Answer from the drawing. Dimensions are ordinates in mm from the lowest x, y and z of the part. A direction names the side the tool comes from. Round coordinates to 2 decimals unless told otherwise and drop trailing zeros. Write each loop counter-clockwise with the first axis right and the second up, starting at its lowest first coordinate (ties: lowest second). Pieces come first, ordered by that corner, then holes.
1. Find section C-C (y = 5.75). Write down the section's boundary in (x, z) (3 decimals).
2. Find section D-D (y = 23.75). Write down the section's boundary in (x, z) (3 decimals), and give its area (3 significant figures).
3. Find section B-B (z = 14). Write down the section's boundary in (x, y), and give its area (3 significant figures).
4. Determine the mould class of the marked faces 3, 4 and 5 for opening direction Z: pulls with the +Z half, pulls with the -Z half, needs draft (parallel to the pull), parting line crosses it, or undercut.
5. Straight lines are drawn through the part: probe 1 along Y at (x, z) = (18, 2); probe 2 along X at (y, z) = (14.5, 16.5); probe 3 along Z at (x, y) = (16, 20). For each, find the intervals that lie inside material, in ascending order.
6. A tool of negligible diameter and unlimited length cuts with its end or side. For the marked faces 1 and 2, from which of +Z, -Z, +X, -X, +Y, -Y can it reach the whole face along a straight path? Write none if from no direction.
7. Find section A-A (x = 22). Write down the section's boundary in (y, z), and give its area (3 significant figures).
8. Flat-ended cylindrical pins translate along their axes: pin 1 Ø2 at (x, y) = (7.5, 18) entering from +Z; pin 2 Ø1.5 at (x, y) = (13.5, 3.5) entering from +Z; pin 3 Ø2 at (x, y) = (14, 13.5) entering from -Z. Find the tip coordinate at first contact, or state that the pin passes through.
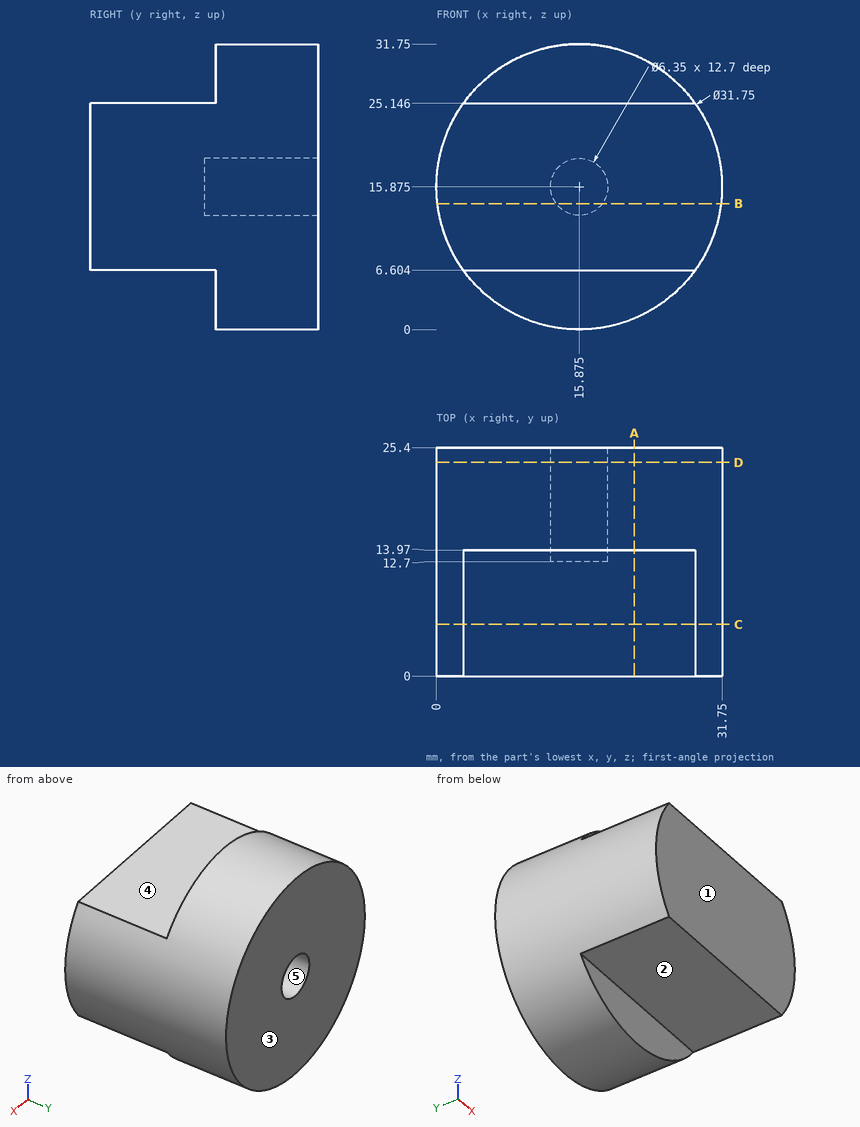
Worked answers:
1. outline: (2.988, 6.604) - (28.762, 6.604) arc R15.875 ccw to (28.762, 25.146) - (2.988, 25.146) arc R15.875 ccw to start
2. outline: circle Ø31.75 at (15.875, 15.875); hole circle Ø6.35 at (15.875, 15.875)
2. area: 760 mm2
3. outline: (0.11, 0) - (31.64, 0) - (31.64, 25.4) - (18.44, 25.4) - (18.44, 12.7) - (13.31, 12.7) - (13.31, 25.4) - (0.11, 25.4) - close
3. area: 736 mm2
4. face 3: needs draft
4. face 4: pulls with the +Z half
4. face 5: undercut
5. probe 1: y = 13.97 to 25.4
5. probe 2: x = 0.01 to 12.76, 18.99 to 31.74
5. probe 3: z = 0 to 12.7, 19.05 to 31.75
6. face 1: +Z, -Z, +X, -X, -Y
6. face 2: -Z, +X, -X, -Y
7. outline: (0, 6.6) - (13.97, 6.6) - (13.97, 1.23) - (25.4, 1.23) - (25.4, 30.52) - (13.97, 30.52) - (13.97, 25.15) - (0, 25.15) - close
7. area: 594 mm2
8. pin 1: stops at z = 29.93
8. pin 2: stops at z = 25.15
8. pin 3: stops at z = 0.03
